Check sheet for the modelled part. Datum: model origin and axes. Units: mm. Coordinates: 2 decimals unless noted, no trailing zeros. Loops run counter-clockwise (first coordinate to the right, second up) from the corner with the lowest first, then second, coordinate; pieces in that order, holes last. Notation, with made-up numbers: (-28.75, 34.5) -> (21.25, 34.5) arc R15 cw to (21.25, 39.5) -> close; hole circle Ø4 at (78.5, 75). An arc over 180 degrees is marked (long way). Use CSV: the item, a comma, the result in double quotes. Start each with the question number.
1. Gauge pin test, flat ends, axial feed: pin 1 (1.2 mm diameter, centred on x = 8, z = 35, fed in from -Y); pin 2 (5 mm diameter, centred on x = 0.5, z = -2, fed in from +Y); pin 3 (1.5 mm diameter, centred on x = -8, y = 4, fed in from +Z). Record the tip position at first contact, or that the pin passes through.
2. Sectioned sample at A-A, the plane z = -5.5. Record the cut outline in (x, y), and give its area (3 significant figures).
3. Sectioned sample at B-B, the plane x = 0. Record the cut outline in (y, z), and give its area (3 significant figures).
4. Sectioned sample at C-C, the plane x = -22. Record the cut outline in (y, z), and give its area (3 significant figures).
5. Thickness scan on L1, parallel to Z at x = 0, y = 1.55; L2, parallel to X at y = 6.5, z = -16.5; L3, parallel to Z at x = -22, y = 6. Record the ranges inside material, lowest first.
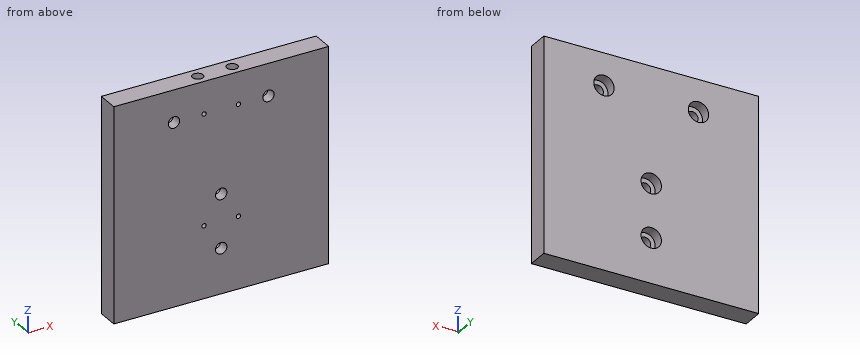
```python
from build123d import *

# Parameters (mm, degrees)
SKETCH_1_W                   = 100
SKETCH_1_H                   = 100
EXTRUDE_1_DEPTH              = 10
HOLE_WIZARD_M2_1_D           = 3
HOLE_WIZARD_M2_1_DEPTH       = 70
HOLE_WIZARD_M2_1_CBORE_D     = 5
HOLE_WIZARD_M2_1_CBORE_DEPTH = 10
HOLE_WIZARD_M5_1_D           = 5.3
HOLE_WIZARD_M5_1_CBORE_D     = 9.5
HOLE_WIZARD_M5_1_CBORE_DEPTH = 5
HOLE_WIZARD_M2_2_D           = 2
HOLE_WIZARD_M2_2_DEPTH       = 8


with BuildPart() as part:
    # 스케치1 → 보스-돌출1 (new body)
    with BuildSketch(Plane(origin=(0, 0, 0), x_dir=(1, 0, 0), z_dir=(0, 1, 0))):
        Rectangle(SKETCH_1_W, SKETCH_1_H)
    extrude(amount=EXTRUDE_1_DEPTH)

    # M2 소켓 머리 캡 나사용 카운터보어1
    with Locations(Plane.XY.offset(50)):
        with Locations((-8, 5), (8, 5)):
            CounterBoreHole(HOLE_WIZARD_M2_1_D / 2, HOLE_WIZARD_M2_1_CBORE_D / 2, HOLE_WIZARD_M2_1_CBORE_DEPTH, depth=HOLE_WIZARD_M2_1_DEPTH)

    # M5 소켓 머리 캡 나사용 카운터보어1 (through all)
    with Locations(Plane(origin=(0, 10, 0), x_dir=(1, 0, 0), z_dir=(0, 1, 0))):
        with Locations((0, 29), (0, 4), (-22, -35), (22, -35)):
            CounterBoreHole(HOLE_WIZARD_M5_1_D / 2, HOLE_WIZARD_M5_1_CBORE_D / 2, HOLE_WIZARD_M5_1_CBORE_DEPTH)

    # M2 여유 구멍2
    with Locations(Plane(origin=(0, 0, 0), x_dir=(-1, 0, 0), z_dir=(0, -1, 0))):
        with Locations((-8, -35), (8, -35), (8, 16.5), (-8, 16.5)):
            Hole(HOLE_WIZARD_M2_2_D / 2, depth=HOLE_WIZARD_M2_2_DEPTH)


solid = part.part
```
Completed:
1,pin 1,"y = 8"
1,pin 2,"y = 5"
1,pin 3,"z = 40"
2,outline,"(-50, 0) -> (-2.18, 0) -> (-2.18, 5) -> (-4.51, 5) -> (-4.51, 10) -> (-50, 10) -> close; (2.18, 0) -> (50, 0) -> (50, 10) -> (4.51, 10) -> (4.51, 5) -> (2.18, 5) -> close; hole circle Ø3 at (-8, 5); hole circle Ø3 at (8, 5)"
2,area,"919 mm²"
3,outline,"(0, -50) -> (10, -50) -> (10, -33.75) -> (5, -33.75) -> (5, -31.65) -> (0, -31.65) -> close; (0, -26.35) -> (5, -26.35) -> (5, -24.25) -> (10, -24.25) -> (10, -8.75) -> (5, -8.75) -> (5, -6.65) -> (0, -6.65) -> close; (0, -1.35) -> (5, -1.35) -> (5, 0.75) -> (10, 0.75) -> (10, 50) -> (0, 50) -> close"
3,area,"852 mm²"
4,outline,"(0, -50) -> (10, -50) -> (10, 30.25) -> (5, 30.25) -> (5, 32.35) -> (0, 32.35) -> close; (0, 37.65) -> (5, 37.65) -> (5, 39.75) -> (10, 39.75) -> (10, 50) -> (0, 50) -> close"
4,area,"926 mm²"
5,L1,"-50 to -31.65, -26.35 to -6.65, -1.35 to 50"
5,L2,"-50 to -9, -7 to 7, 9 to 50"
5,L3,"-50 to 30.25, 39.75 to 50"
